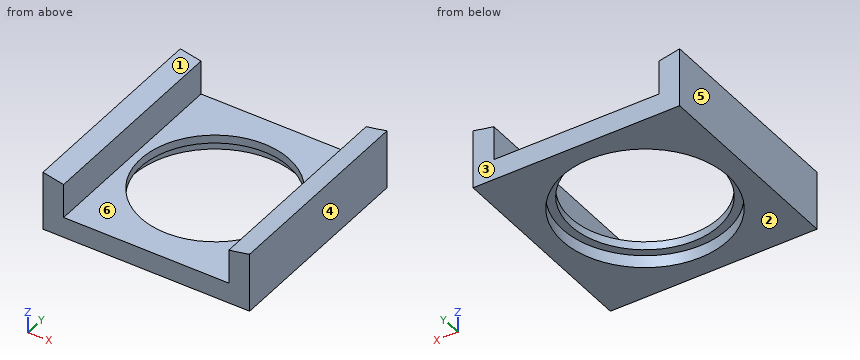
```python
from build123d import *

# Parameters (mm, degrees)
SKETCH2_W               = 50
SKETCH2_H               = 50
BOSS_EXTRUDE1_DEPTH     = 5
SKETCH3_W               = 5
SKETCH3_H               = 50
SKETCH3_W_2             = 5.036023039
BOSS_EXTRUDE2_DEPTH     = 11
CUT_EXTRUDE3_DEPTH      = 51.174718111
CUT_EXTRUDE3_DEPTH_BACK = 51.174718111
SKETCH5_R               = 18
SKETCH6_R               = 20
CUT_EXTRUDE4_DEPTH      = 3
CUT_EXTRUDE5_DEPTH      = 51.174718111
CUT_EXTRUDE5_DEPTH_BACK = 51.174718111
SKETCH7_R               = 112.5


with BuildPart() as part:
    # Sketch2 → Boss-Extrude1 (new body)
    with BuildSketch(Plane.XY):
        with Locations((-12.301587302, 4.497354497)):
            Rectangle(SKETCH2_W, SKETCH2_H)
    extrude(amount=BOSS_EXTRUDE1_DEPTH)

    # Sketch3 → Boss-Extrude2 (add)
    with BuildSketch(Plane.XY.offset(5)):
        with Locations((-34.801587302, 4.497354497)):
            Rectangle(SKETCH3_W, SKETCH3_H)
        with Locations((10.180401179, 4.497354497)):
            Rectangle(SKETCH3_W_2, SKETCH3_H)
    extrude(amount=BOSS_EXTRUDE2_DEPTH)

    # Sketch5 → Cut-Extrude3 (cut, two sides: drawn at the far end of the back side and taken through both)
    with BuildSketch(Plane.XY.offset(-CUT_EXTRUDE3_DEPTH_BACK)):
        with Locations((-12.319598821, 4.529496056)):
            Circle(SKETCH5_R)
    extrude(amount=CUT_EXTRUDE3_DEPTH + CUT_EXTRUDE3_DEPTH_BACK, mode=Mode.SUBTRACT)

    # Sketch6 → Cut-Extrude4 (cut)
    with BuildSketch(Plane(origin=(0, 0, 0), x_dir=(-1, 0, 0), z_dir=(0, 0, -1))):
        with Locations((12.319598821, 4.529496056)):
            Circle(SKETCH6_R)
    extrude(amount=-CUT_EXTRUDE4_DEPTH, mode=Mode.SUBTRACT)

    # Sketch7 → Cut-Extrude5 (cut, two sides: drawn at the far end of the back side and taken through both)
    with BuildSketch(Plane(origin=(0, 0, 0), x_dir=(1, 0, 0), z_dir=(0, 1, 0)).offset(-CUT_EXTRUDE5_DEPTH_BACK)):
        with Locations((-12.319598821, -124)):
            Circle(SKETCH7_R)
    extrude(amount=CUT_EXTRUDE5_DEPTH + CUT_EXTRUDE5_DEPTH_BACK, mode=Mode.SUBTRACT)


solid = part.part
```
For this review, take the finished solid that the model builds, in its own axes (mm). Face numbers are marked on the shaded views. A direction names the side the tool comes from. Coordinates: 2 decimals unless noted, no trailing zeros. Write each loop counter-clockwise with the first axis right and the second up, starting at its lowest first coordinate (ties: lowest second). Pieces come first, ordered by that corner, then holes. Notation, with made-up numbers: (82.25, -30) - (91.25, -30) arc R24 cw to (91.25, -15) - close; hole circle Ø11 at (31.25, 26.25). An arc over 180 degrees is marked (long way). Answer in a Markdown table with one row per item. Add a question column.
Q1. For P1, Ø20, axis at x = -9.5, y = 13, coming from the +Z side; P2, Ø8, axis at x = 7, z = 11.5, coming from the -Y side, all flat-tipped, find the tip position at first contact; note any pin that passes through.
Q2. We need section D-D, the plane y = -12. State the section outline as (x, z) points.
Q3. Draft analysis for pull direction X (two halves, no side actions). For the marked faces 3, 4, 5 and 6, state which applies: +X half, -X half, draft (parallel to the pull), parting line (faces both ways), or undercut.
Q4. We need section A-A, the plane z = 11.25. State the section outline as (x, y) points, and give its area (3 significant figures).
Q5. Tool access review of the marked faces 1 and 2: name each direction out of +Z, -Z, +X, -X, +Y, -Y from which nothing blocks a thin tool from reaching the whole face with its end or side.
Q6. We need section B-B, the plane y = 13.5. State the section outline as (x, z) points (3 decimals).
Q7. For probe 1 along X at (y, z) = (-13, 10.5); probe 2 along Z at (x, y) = (7, 20); probe 3 along Y at (x, z) = (-13.5, 1.75), list the stretches that pass through material, from the lowest coordinate up.
Q8. We need section C-C, the plane x = -21. State the section outline as (y, z) points, and give its area (3 significant figures).
Answer list:
| question | item | result |
|---|---|---|
| 1 | P1 | stops at z = 5 |
| 1 | P2 | stops at y = -20.5 |
| 2 | outline | (-37.3, 0) - (-23.58, 0) - (-23.58, 3) - (-19.45, 3) - (-19.45, 5) - (-32.3, 5) - (-32.3, 13.29) arc R112.5 cw to (-37.3, 14.31) - close; (-5.19, 3) - (-1.06, 3) - (-1.06, 0) - (12.7, 0) - (12.7, 14.32) arc R112.5 cw to (7.66, 13.29) - (7.66, 5) - (-5.19, 5) - close |
| 3 | face 3 | draft |
| 3 | face 4 | +X half |
| 3 | face 5 | -X half |
| 3 | face 6 | undercut |
| 4 | outline | (-37.3, -20.5) - (-32.3, -20.5) - (-32.3, 29.5) - (-37.3, 29.5) - close; (7.66, -20.5) - (12.7, -20.5) - (12.7, 29.5) - (7.66, 29.5) - close |
| 4 | area | 502 mm2 |
| 5 | face 1 | +Z, +Y, -Y |
| 5 | face 2 | -Z, +X, -X, +Y, -Y |
| 6 | outline | (-37.302, 0) - (-30.195, 0) - (-30.195, 3) - (-27.925, 3) - (-27.925, 5) - (-32.302, 5) - (-32.302, 13.289) arc R112.5 cw to (-37.302, 14.309) - close; (3.286, 3) - (5.556, 3) - (5.556, 0) - (12.698, 0) - (12.698, 14.317) arc R112.5 cw to (7.662, 13.289) - (7.662, 5) - (3.286, 5) - close |
| 7 | probe 1 | x = -37.3 to -32.3, 7.66 to 12.7 |
| 7 | probe 2 | z = 0 to 5 |
| 7 | probe 3 | y = -20.5 to -15.44, 24.49 to 29.5 |
| 8 | outline | (-20.5, 0) - (-13.49, 0) - (-13.49, 3) - (-11.24, 3) - (-11.24, 5) - (-20.5, 5) - close; (20.3, 3) - (22.55, 3) - (22.55, 0) - (29.5, 0) - (29.5, 5) - (20.3, 5) - close |
| 8 | area | 78.8 mm2 |
